Drawing for the job (mm, zero at the part's lowest x, y, z). Give positions to 0.01 mm unless a question says otherwise; leave off trailing zeros. Order: outer loops, then holes, each group sorted by start corner. A loop starts at its lowest first (then second) coordinate and runs counter-clockwise, first axis right, second up. Notation, with made-up numbers: M 55.25,42 L 104.25,42 A27 cw 104.25,62 Z; hole C 38,-17.5 d11. An arc over 180 degrees is marked long. Answer as a JSON object with one key per item and string values.
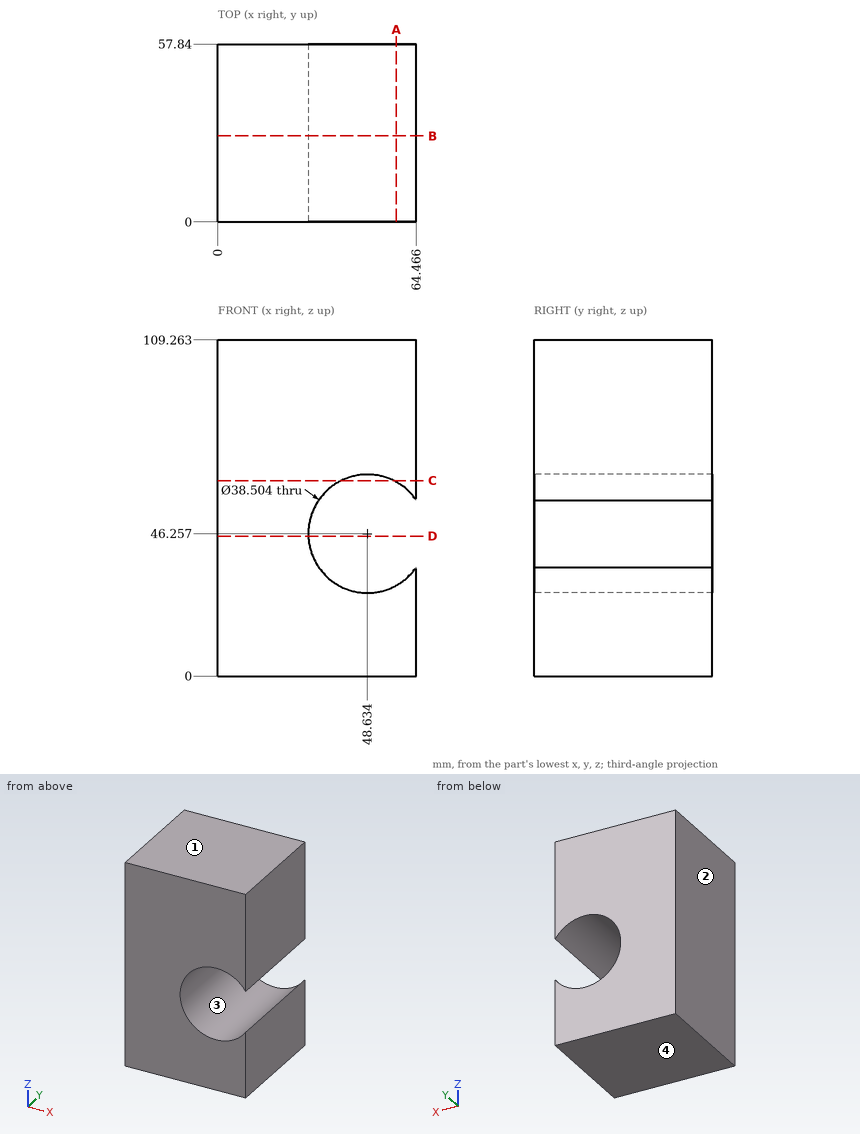
1. Cut at A-A on x = 58. Give the cut face in (y, z), plus the area to 3 significant figures.
Worked answers:
{"outline": "M 0,0 L 57.84,0 L 57.84,29.44 L 0,29.44 Z; M 0,63.08 L 57.84,63.08 L 57.84,109.26 L 0,109.26 Z", "area": "4,370 mm^2"}
2. Cut at C-C on z = 63.5. Give the cut face in (x, y), plus the area to 3 significant figures.
Worked answers:
{"outline": "M 0,0 L 40.07,0 L 40.07,57.84 L 0,57.84 Z; M 57.2,0 L 64.47,0 L 64.47,57.84 L 57.2,57.84 Z", "area": "2,740 mm^2"}
3. Pin check, flat tip, straight feed: P1, Ø3, axis at x = 32, y = 9.5, coming from the -Z side. Stop position of the tip, or through.
Worked answers:
{"P1": "stops at z = 0"}
4. Two-plate mould, pull along Z, no slides. Class the marked faces 1, 2, 3 and 4: +Z half, -Z half, draft (parallel to the pull), parting line (faces both ways), or undercut.
Worked answers:
{"face 1": "+Z half", "face 2": "draft", "face 3": "undercut", "face 4": "-Z half"}
5. Cut at D-D on z = 45.5. Give the cut face in (x, y), plus the area to 3 significant figures.
Worked answers:
{"outline": "M 0,0 L 29.4,0 L 29.4,57.84 L 0,57.84 Z", "area": "1,700 mm^2"}
6. Cut at B-B on y = 28. Give the cut face in (x, z), plus the area to 3 significant figures.
Worked answers:
{"outline": "M 0,0 L 64.47,0 L 64.47,35.3 A19.25 cw long 64.47,57.21 L 64.47,109.26 L 0,109.26 Z", "area": "5,930 mm^2"}
7. Probe line 1 along Z through (x, y) = (33, 29.5) (1 decimal); line 2 along Z through (x, y) = (41, 35); line 3 along X through (y, z) = (6, 32) (1 decimal). List the from-to ranges inside material, lowest first.
Worked answers:
{"line 1": "z = 0 to 35, 57.5 to 109.3", "line 2": "z = 0 to 28.58, 63.93 to 109.26", "line 3": "x = 0 to 35.7, 61.6 to 64.5"}
